```python
from build123d import *

# Parameters (mm, degrees)
F0_R     = 9.525
F1_DEPTH = 38.1
F2_W     = 6.35
F2_H     = 6.35
F3_DEPTH = 12.7
F4_W     = 94.41996
F4_H     = 25.4
F5_DEPTH = 44.45


with BuildPart() as f1:
    # F0 (on Front) → F1 (new body)
    with BuildSketch(Plane.XZ):
        Polygon((-396.128201, 181.143697), (-415.178201, 181.143697), (-415.178201, 143.043697), (-323.230201, 143.043697), (-341.951291, 175.469577), (-373.776201, 193.843697), (-396.128201, 193.843697), align=None)
        with Locations((-377.078201, 168.443697)):
            Circle(F0_R, mode=Mode.SUBTRACT)
    extrude(amount=F1_DEPTH)

    # F2 (on face) → F3 (join)
    with BuildSketch(Plane.XY.offset(181.143697)):
        with Locations((-405.653201, -9.525)):
            Rectangle(F2_W, F2_H)
    extrude(amount=F3_DEPTH)

    # F4 (on face) → F5 (cut)
    with BuildSketch(Plane.XY.offset(193.843697)):
        with Locations((-361.618221, -19.05)):
            Rectangle(F4_W, F4_H)
    extrude(amount=-F5_DEPTH, mode=Mode.SUBTRACT)


solid = f1.part
```
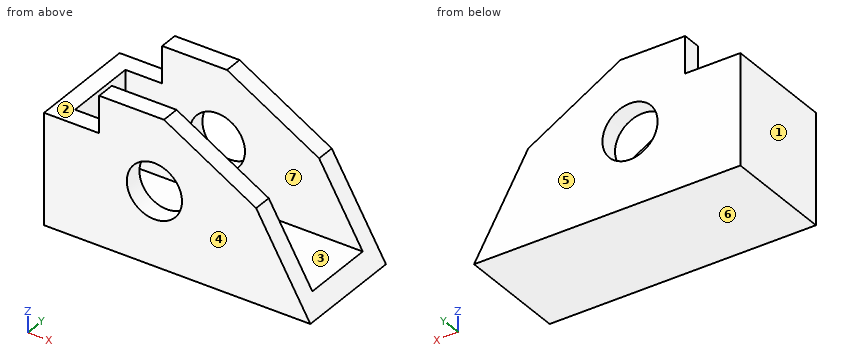
Model file for the job. Use its own axes, mm. Face numbers are marked on the shaded views. A direction names the side the tool comes from. Coordinates: 2 decimals unless noted, no trailing zeros. Order: outer loops, then holes, each group sorted by start corner. A loop starts at its lowest first (then second) coordinate and runs counter-clockwise, first axis right, second up. Notation, with made-up numbers: (29.5, 4) -> (36.5, 4) arc R18 cw to (36.5, 25) -> close; hole circle Ø1 at (86.5, 75.25). An arc over 180 degrees is marked (long way). Answer as a JSON object with one key per item and string values. Group by question number.
1) Cut at D-D, the plane x = -351. Write the cut outline in (y, z), then the cut area to 3 significant figures.
2) Cut at B-B, the plane z = 190. Write the cut outline in (x, y).
3) Flat gauge pins, fed straight in: pin 1 (7.5 mm diameter, centred on y = -24.5, z = 169.5, fed in from +X); pin 2 (7 mm diameter, centred on y = -34, z = 186.5, fed in from -X); pin 3 (7.5 mm diameter, centred on x = -355, y = -18.5, fed in from +Z); pin 4 (6 mm diameter, centred on y = -15.5, z = 184.5, fed in from +X). Where does each tip first touch, or does it go through?
4) Which spindle directions (+Z, -Z, +X, -X, +Y, -Y) get a long thin tool onto all of the face, cutting with end or side? Do the marked faces 1, 2 and 3. Say none if no direction does.
5) Drill centre lines: L1, parallel to Y at x = -346.5, z = 162; L2, parallel to Z at x = -379.5, y = -19; L3, parallel to X at y = -24.5, z = 171. Where is each one in solid material? Low to high.
6) Pull direction Y, two halves, no side cores. Call the marked faces 4, 5, 6 and 7: +Y half, -Y half, draft (parallel to the pull), parting line (faces both ways), or undercut.
7) Cut at A-A, the plane z = 166.5. Write the cut outline in (x, y).
8) Cut at C-C, the plane y = -27. Write the cut outline in (x, z), then the cut area to 3 significant figures.
Check values:
{
 "1": {"outline": "(-38.1, 143.04) -> (0, 143.04) -> (0, 180.69) -> (-6.35, 180.69) -> (-6.35, 149.39) -> (-31.75, 149.39) -> (-31.75, 180.69) -> (-38.1, 180.69) -> close", "area": "639 mm²"},
 "2": {"outline": "(-396.13, -38.1) -> (-367.12, -38.1) -> (-367.12, -31.75) -> (-396.13, -31.75) -> close; (-396.13, -6.35) -> (-367.12, -6.35) -> (-367.12, 0) -> (-396.13, 0) -> close"},
 "3": {"pin 1": "stops at x = -408.83", "pin 2": "stops at x = -396.13", "pin 3": "stops at z = 149.39", "pin 4": "passes through"},
 "4": {"face 1": "+Z, -Z, -X, +Y, -Y", "face 2": "+Z, -X, +Y, -Y", "face 3": "+Z, +X"},
 "5": {"L1": "y = -38.1 to -31.75, -6.35 to 0", "L2": "z = 143.04 to 149.39", "L3": "x = -415.18 to -408.83"},
 "6": {"face 4": "-Y half", "face 5": "+Y half", "face 6": "draft", "face 7": "undercut"},
 "7": {"outline": "(-415.18, -38.1) -> (-386.4, -38.1) -> (-386.4, -31.75) -> (-408.83, -31.75) -> (-408.83, -6.35) -> (-386.4, -6.35) -> (-386.4, 0) -> (-415.18, 0) -> close; (-367.75, -38.1) -> (-336.77, -38.1) -> (-336.77, -31.75) -> (-367.75, -31.75) -> close; (-367.75, -6.35) -> (-336.77, -6.35) -> (-336.77, 0) -> (-367.75, 0) -> close"},
 "8": {"outline": "(-415.18, 143.04) -> (-323.23, 143.04) -> (-326.9, 149.39) -> (-408.83, 149.39) -> (-408.83, 181.14) -> (-415.18, 181.14) -> close", "area": "774 mm²"}
}
